The drawing under review shows one solid part. Ordinate dimensions are in mm from its lowest x, y, z. A direction names the side the tool comes from. Give positions to 0.01 mm unless a question says otherwise; leave off trailing zeros. Loops run counter-clockwise (first coordinate to the right, second up) from the corner with the lowest first, then second, coordinate; pieces in that order, holes last. Notation, with made-up numbers: M 70.25,79 L 96.25,79 A15 ccw 96.25,84 Z; hole C 19.25,42.5 d3. An arc over 180 degrees is marked long. Put each result on its own line as item: value. Start each with the question number.
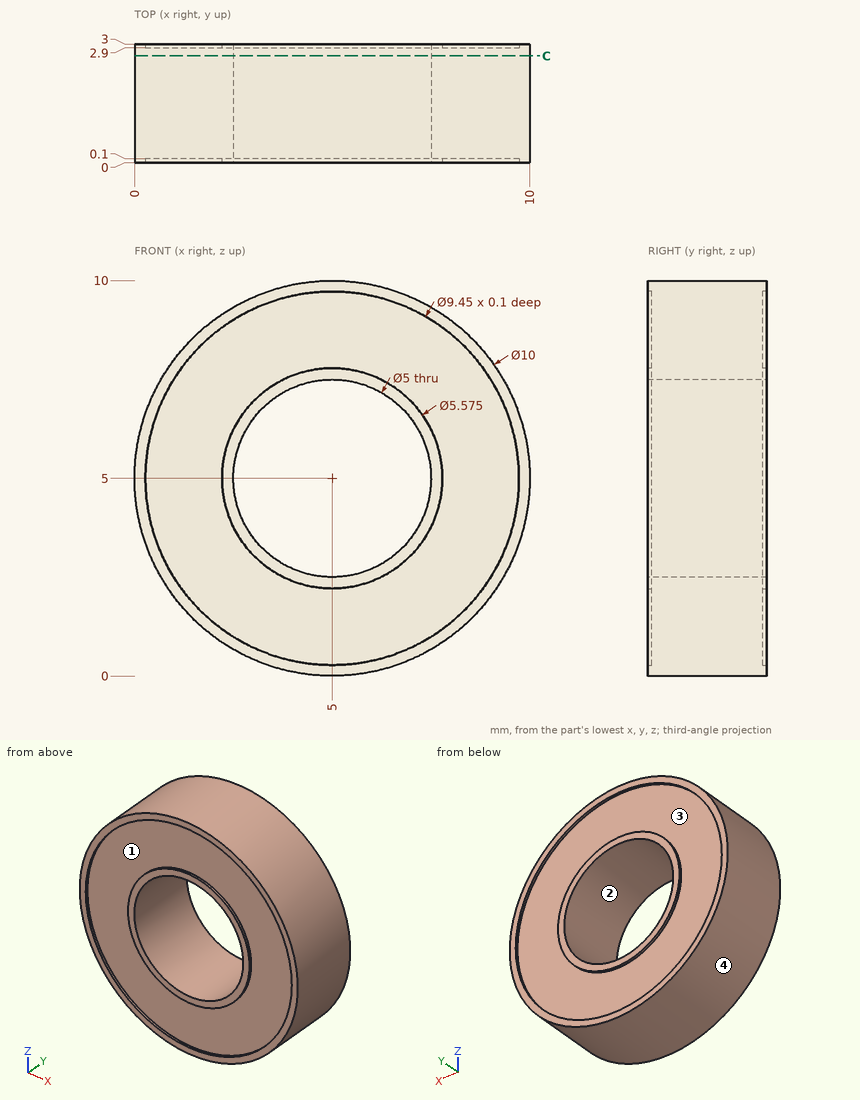
Item 1: Tool access review of the marked faces 1 and 2: name each direction out of +Z, -Z, +X, -X, +Y, -Y from which nothing blocks a thin tool from reaching the whole face with its end or side.
Item 2: Clearance check with flat-ended pins moving along their axes: pin 1 Ø1 at (x, y) = (3, 1) entering from +Z; pin 2 Ø3 at (x, z) = (3, 5.5) entering from +Y; pin 3 Ø1 at (x, y) = (8, 1) entering from +Z. State where each tip first meets the part, or that it passes through.
Item 3: To check wall thickness, follow L1, parallel to X at y = 0.05, z = 5 (1 decimal); L2, parallel to X at y = 0.95, z = 5; L3, parallel to Y at x = 2.5, z = 6.75. State the ranges of each line that lie inside material, in increasing order. Write a range as [from, to].
Item 4: Consider section C-C, the plane y = 2.7. Write out the cut boundary in (x, z), plus the area to 3 significant figures.
Item 5: Draft analysis for pull direction Z (two halves, no side actions). For the marked faces 3 and 4, state which applies: +Z half, -Z half, draft (parallel to the pull), parting line (faces both ways), or undercut.
Report:
1. face 1: -Y
1. face 2: +Y, -Y
2. pin 1: z = 9.77
2. pin 2: y = 3
2. pin 3: z = 9.33
3. L1: [0, 0.3], [2.2, 2.5], [7.5, 7.8], [9.7, 10]
3. L2: [0, 2.5], [7.5, 10]
3. L3: [0.1, 2.9]
4. outline: C 5,5 d10; hole C 5,5 d5
4. area: 58.9 mm²
5. face 3: undercut
5. face 4: parting line
